Input: dimensioned drawing with shaded views. Units: mm. Origin: part minimum x, y, z. Give positions to 0.01 mm unless a question says otherwise; leave off trailing zeros. Write each loop counter-clockwise with the first axis right and the second up, starting at its lowest first coordinate (ties: lowest second). Pieces come first, ordered by that corner, then holes. Notation, with made-up numbers: (-3, -7.5) - (21, -7.5) arc R15 ccw to (21, 13.5) - close; hole circle Ø1 at (-18.75, -32.75). An arc over 180 degrees is marked (long way). Answer as a JSON object with one key per item and string values. Group by question number.
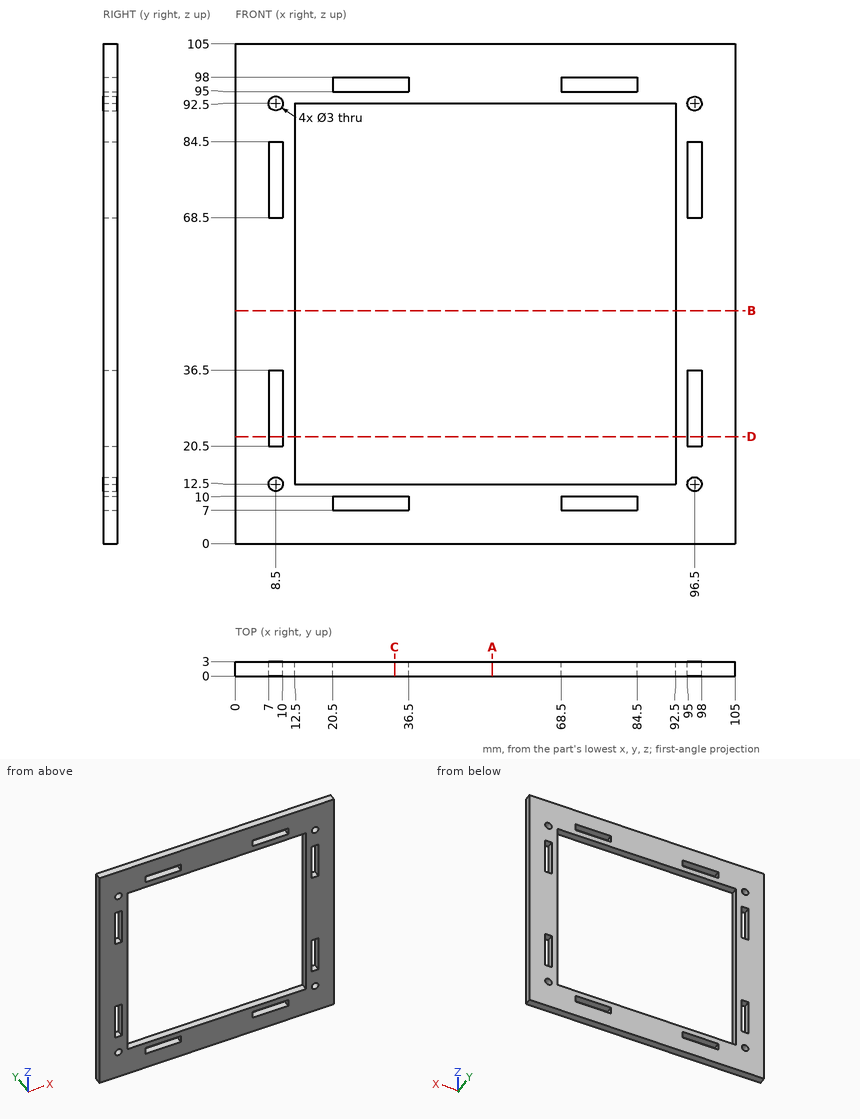
1) Pin query (flat end, axial travel): P1, Ø2.5, axis at x = 96.5, z = 92.5, coming from the -Y side. Return the tip coordinate at first contact, or that it passes through.
2) Cut plane A-A on x = 54. Return the cut outline in (y, z).
3) Cut plane B-B on z = 49. Return the cut outline in (x, y), and give its area (3 significant figures).
4) Cut plane D-D on z = 22.5. Return the cut outline in (x, y).
5) Line query: line 1 along X through (y, z) = (0.75, 22.5); line 2 along X through (y, z) = (0.55, 61.5). Output: solid intervals per line, ascending. Write a range as from..to.
6) Cut plane C-C on x = 33.5. Return the cut outline in (y, z).
Filled in:
{
 "1": {"P1": "passes through"},
 "2": {"outline": "(0, 0) - (3, 0) - (3, 12.5) - (0, 12.5) - close; (0, 92.5) - (3, 92.5) - (3, 105) - (0, 105) - close"},
 "3": {"outline": "(0, 0) - (12.5, 0) - (12.5, 3) - (0, 3) - close; (92.5, 0) - (105, 0) - (105, 3) - (92.5, 3) - close", "area": "75.0 mm²"},
 "4": {"outline": "(0, 0) - (7, 0) - (7, 3) - (0, 3) - close; (10, 0) - (12.5, 0) - (12.5, 3) - (10, 3) - close; (92.5, 0) - (95, 0) - (95, 3) - (92.5, 3) - close; (98, 0) - (105, 0) - (105, 3) - (98, 3) - close"},
 "5": {"line 1": "x = 0..7, 10..12.5, 92.5..95, 98..105", "line 2": "x = 0..12.5, 92.5..105"},
 "6": {"outline": "(0, 0) - (3, 0) - (3, 7) - (0, 7) - close; (0, 10) - (3, 10) - (3, 12.5) - (0, 12.5) - close; (0, 92.5) - (3, 92.5) - (3, 95) - (0, 95) - close; (0, 98) - (3, 98) - (3, 105) - (0, 105) - close"}
}
